```python
from build123d import *

# Parameters (mm, degrees)
SKETCH1_R           = 2
BOSS_EXTRUDE1_DEPTH = 2
SKETCH2_W           = 2.8
SKETCH2_H           = 27
BOSS_EXTRUDE2_DEPTH = 10
SKETCH3_R           = 1.5
CUT_EXTRUDE1_DEPTH  = 114.824325613
FILLET1_R           = 1.5
FILLET2_R           = 2


with BuildPart() as part:
    # Sketch1 → Boss-Extrude1 (new body)
    with BuildSketch(Plane(origin=(0, 0, 0), x_dir=(1, 0, 0), z_dir=(0, 1, 0))):
        Polygon((0, 6), (2, 0), (33, 0), (35, 5.5), (66, 5.5), (68, 0), (99, 0), (101, 6), (101, 39.094975397), (0, 39.094975397), align=None)
        with Locations(Location((9.5, 5.5, 0), (0, 0, 270))):
            Circle(SKETCH1_R, mode=Mode.SUBTRACT)
        with Locations(Location((23.5, 5.5, 0), (0, 0, 270))):
            Circle(SKETCH1_R, mode=Mode.SUBTRACT)
        with Locations(Location((77.5, 5.5, 0), (0, 0, 90))):
            Circle(SKETCH1_R, mode=Mode.SUBTRACT)
        with Locations(Location((91.5, 5.5, 0), (0, 0, 90))):
            Circle(SKETCH1_R, mode=Mode.SUBTRACT)
        with Locations(Location((30, 23.149785568, 0), (0, 0, 270))):
            Circle(SKETCH1_R, mode=Mode.SUBTRACT)
        with Locations(Location((38, 23.149785568, 0), (0, 0, 270))):
            Circle(SKETCH1_R, mode=Mode.SUBTRACT)
        with Locations(Location((63, 23.149785568, 0), (0, 0, 90))):
            Circle(SKETCH1_R, mode=Mode.SUBTRACT)
        with Locations(Location((71, 23.149785568, 0), (0, 0, 90))):
            Circle(SKETCH1_R, mode=Mode.SUBTRACT)
        Polygon((11, 22.094975397), (14, 19.094975397), (22, 19.094975397), (22, 27.094975397), (11, 27.094975397), align=None, mode=Mode.SUBTRACT)
        Polygon((90, 27.094975397), (90, 22.094975397), (87, 19.094975397), (79, 19.094975397), (79, 27.094975397), align=None, mode=Mode.SUBTRACT)
    extrude(amount=BOSS_EXTRUDE1_DEPTH)

    # Sketch2 → Boss-Extrude2 (add)
    with BuildSketch(Plane(origin=(0, 2, 0), x_dir=(1, 0, 0), z_dir=(0, 1, 0))):
        with Locations((-1.4, 23.094975397)):
            Rectangle(SKETCH2_W, SKETCH2_H)
        with Locations((102.4, 23.094975397)):
            Rectangle(SKETCH2_W, SKETCH2_H)
    extrude(amount=-BOSS_EXTRUDE2_DEPTH)

    # Sketch3 → Cut-Extrude1 (cut, through all)
    with BuildSketch(Plane(origin=(103.8, 0, 0), x_dir=(0, 0, -1), z_dir=(1, 0, 0))):
        with Locations((13.094975397, -4.5)):
            Circle(SKETCH3_R)
        with Locations((32.094975397, -4.5)):
            Circle(SKETCH3_R)
    extrude(amount=-CUT_EXTRUDE1_DEPTH, mode=Mode.SUBTRACT)

    # Fillet1
    fillet1_edges = [part.edges().sort_by_distance(p)[0] for p in [
        (-1.4, -8, -9.594975397),
        (-1.4, -8, -36.594975397),
        (0, 1, -9.594975397),
        (0, 1, -6),
        (2, 1, 0),
        (0, 1, -36.594975397),
        (102.4, -8, -36.594975397),
        (101, 1, -36.594975397),
        (102.4, -8, -9.594975397),
        (101, 1, -9.594975397),
        (101, 1, -6),
        (99, 1, 0),
        (66, 1, -5.5),
        (68, 1, 0),
        (90, 1, -27.094975397),
        (79, 1, -27.094975397),
        (90, 1, -22.094975397),
        (87, 1, -19.094975397),
        (79, 1, -19.094975397),
        (35, 1, -5.5),
        (33, 1, 0),
        (11, 1, -27.094975397),
        (11, 1, -22.094975397),
        (14, 1, -19.094975397),
        (22, 1, -19.094975397),
        (22, 1, -27.094975397),
    ]]
    fillet(fillet1_edges, radius=FILLET1_R)

    # Fillet2
    fillet2_edges = [part.edges().sort_by_distance(p)[0] for p in [
        (-2.8, 2, -23.094975397),
        (103.8, 2, -23.094975397),
    ]]
    fillet(fillet2_edges, radius=FILLET2_R)


solid = part.part
```
Model file for the job. Use its own axes, mm. A direction names the side the tool comes from. Coordinates: 2 decimals unless noted, no trailing zeros. Loops run counter-clockwise (first coordinate to the right, second up) from the corner with the lowest first, then second, coordinate; pieces in that order, holes last. Notation, with made-up numbers: (72.5, 4) -> (91.5, 4) arc R18 ccw to (91.5, 37) -> close; hole circle Ø2 at (57.5, 78). An arc over 180 degrees is marked (long way). Answer as a JSON object with one key per item and string values.
Q1. Cut at C-C (z = -16.5). List the corners of the cut face in (x, y).
Report:
{"outline": "(-2.8, -8) -> (0, -8) -> (0, 0) -> (101, 0) -> (101, -8) -> (103.8, -8) -> (103.8, 0) arc R2 ccw to (101.8, 2) -> (-0.8, 2) arc R2 ccw to (-2.8, 0) -> close"}
Q2. Probe probe 1 along X at (y, z) = (-6.5, -20.5); probe 2 along Y at (x, z) = (35, -13.5); probe 3 along X at (y, z) = (0.25, -17). List the from-to ranges inside material, lowest first.
Report:
{"probe 1": "x = -2.8 to 0, 101 to 103.8", "probe 2": "y = 0 to 2", "probe 3": "x = -2.78 to 103.78"}
Q3. 3-axis set-ups, long thin cutter, end or side, ignore diameter. For faces 1 (the flat face through (84, 1, -27.095)), 2 (the flat face through (-2.8, -4, -23)), 3 (the flat face through (0, -4, -23)): which of +Z, -Z, +X, -X, +Y, -Y reach the whole face in a straight line?
Report:
{"face 1": "+Y, -Y", "face 2": "+Z, -Z, -X, +Y, -Y", "face 3": "+Z, -Z, -Y"}
Q4. Cut at B-B (y = -1.5). List the corners of the cut face in (x, z), and give its area (3 significant figures).
Report:
{"outline": "(-2.8, -36.59) -> (0, -36.59) -> (0, -9.59) -> (-2.8, -9.59) -> close; (101, -36.59) -> (103.8, -36.59) -> (103.8, -9.59) -> (101, -9.59) -> close", "area": "151 mm2"}
Q5. Cut at A-A (x = 9.5). List the corners of the cut face in (y, z), and give its area (3 significant figures).
Report:
{"outline": "(0, -39.09) -> (2, -39.09) -> (2, -7.5) -> (0, -7.5) -> close; (0, -3.5) -> (2, -3.5) -> (2, 0) -> (0, 0) -> close", "area": "70.2 mm2"}
Q6. Pull direction X, two halves, no side cores. Call faces 4 (the flat face through (101, -4, -23)), 5 (the cylindrical face through (-2.23, 1.4, -23.29)), 6 (the flat face through (103.8, -4, -23)): released by +X, released by -X, zero draft, split by the parting line, or undercut.
Report:
{"face 4": "undercut", "face 5": "released by -X", "face 6": "released by +X"}
Q7. Flat gauge pins, fed straight in: P1, Ø2.5, axis at x = 77.5, z = -5.5, coming from the -Y side; P2, Ø6.5, axis at x = 23.5, z = -5.5, coming from the -Y side; P3, Ø1.4, axis at x = 103, y = -2, coming from the -Z side (3 decimals); P4, Ø1.6, axis at x = 47, y = 1, coming from the +Z side. Where does each tip first touch, or does it go through?
Report:
{"P1": "passes through", "P2": "stops at y = 0", "P3": "stops at z = -36.595", "P4": "stops at z = -5.5"}
